```python
from build123d import *

# Parameters (mm, degrees)
SKETCH1_W           = 140
SKETCH1_H           = 205
SKETCH1_R           = 2.125
BOSS_EXTRUDE1_DEPTH = 3.175
SKETCH2_R           = 2.125
CUT_EXTRUDE1_DEPTH  = 125.162516989


with BuildPart() as part:
    # Sketch1 → Boss-Extrude1 (new body)
    with BuildSketch(Plane.XY):
        Rectangle(SKETCH1_W, SKETCH1_H)
        with Locations((0, 91.5)):
            Circle(SKETCH1_R, mode=Mode.SUBTRACT)
        with Locations((25.11473671, 48)):
            Circle(SKETCH1_R, mode=Mode.SUBTRACT)
        with Locations((-25.11473671, 48)):
            Circle(SKETCH1_R, mode=Mode.SUBTRACT)
        with Locations((0, 62.5)):
            Circle(SKETCH1_R, mode=Mode.SUBTRACT)
        with Locations((-62, -94.5)):
            Circle(SKETCH1_R, mode=Mode.SUBTRACT)
        with Locations(Location((-38, -94.5, 0), (0, 0, 180))):
            Circle(SKETCH1_R, mode=Mode.SUBTRACT)
        with Locations((-38, -70.5)):
            Circle(SKETCH1_R, mode=Mode.SUBTRACT)
        with Locations(Location((-62, -70.5, 0), (0, 0, 180))):
            Circle(SKETCH1_R, mode=Mode.SUBTRACT)
        with Locations((38, -94.5)):
            Circle(SKETCH1_R, mode=Mode.SUBTRACT)
        with Locations(Location((62, -94.5, 0), (0, 0, 180))):
            Circle(SKETCH1_R, mode=Mode.SUBTRACT)
        with Locations((62, -70.5)):
            Circle(SKETCH1_R, mode=Mode.SUBTRACT)
        with Locations(Location((38, -70.5, 0), (0, 0, 180))):
            Circle(SKETCH1_R, mode=Mode.SUBTRACT)
    extrude(amount=BOSS_EXTRUDE1_DEPTH)

    # Sketch2 → Cut-Extrude1 (cut, through all)
    with BuildSketch(Plane.XY.offset(3.175)):
        with Locations((-62, 94.5)):
            Circle(SKETCH2_R)
        with Locations((-62, 60.5)):
            Circle(SKETCH2_R)
        with Locations((-62, 26.5)):
            Circle(SKETCH2_R)
        with Locations((-62, -7.5)):
            Circle(SKETCH2_R)
        with Locations((-28, 26.5)):
            Circle(SKETCH2_R)
        with Locations((-28, -7.5)):
            Circle(SKETCH2_R)
        with Locations(Location((28, -7.5, 0), (0, 0, 180))):
            Circle(SKETCH2_R)
        with Locations(Location((28, 26.5, 0), (0, 0, 180))):
            Circle(SKETCH2_R)
        with Locations(Location((62, -7.5, 0), (0, 0, 180))):
            Circle(SKETCH2_R)
        with Locations(Location((62, 26.5, 0), (0, 0, 180))):
            Circle(SKETCH2_R)
        with Locations(Location((62, 60.5, 0), (0, 0, 180))):
            Circle(SKETCH2_R)
        with Locations(Location((62, 94.5, 0), (0, 0, 180))):
            Circle(SKETCH2_R)
    extrude(amount=-CUT_EXTRUDE1_DEPTH, mode=Mode.SUBTRACT)


solid = part.part
```
Part model, mm, in its own coordinate system. Round coordinates to 2 decimals unless told otherwise and drop trailing zeros. Order: outer loops, then holes, each group sorted by start corner. A loop starts at its lowest first (then second) coordinate and runs counter-clockwise, first axis right, second up. Notation, with made-up numbers: M 19.25,42 L 55.25,42 A34 cw 55.25,75 Z; hole C 77,47.5 d4. An arc over 180 degrees is marked long. Put each result on its own line as item: value. Start each with the question number.
1. Slice it at C-C on y = -7.5. List the corners of the cut face in (x, z) (3 decimals), then the cut area to 3 significant figures.
2. Drop a flat-ended pin along its axis: pin 1 (2.5 mm diameter, centred on x = -62, y = -70.5, fed in from +Z). Give the stop position or say it passes through.
3. Drill centre lines: probe 1 along Y at (x, z) = (-28, 1.95) (3 decimals); probe 2 along X at (y, z) = (59, 2.55); probe 3 along X at (y, z) = (63.5, 1.5) (3 decimals). Where is each one in solid material? Low to high. Write a range as [from, to].
4. Slice it at D-D on x = -38. List the corners of the cut face in (y, z) (3 decimals), then the cut area to 3 significant figures.
5. Slice it at B-B on x = -62. List the corners of the cut face in (y, z) (3 decimals).
6. Slice it at A-A on y = 48. List the corners of the cut face in (x, z) (3 decimals).
Findings:
1. outline: M -70,0 L -64.125,0 L -64.125,3.175 L -70,3.175 Z; M -59.875,0 L -30.125,0 L -30.125,3.175 L -59.875,3.175 Z; M -25.875,0 L 25.875,0 L 25.875,3.175 L -25.875,3.175 Z; M 30.125,0 L 59.875,0 L 59.875,3.175 L 30.125,3.175 Z; M 64.125,0 L 70,0 L 70,3.175 L 64.125,3.175 Z
1. area: 391 mm2
2. pin 1: through
3. probe 1: [-102.5, -9.625], [-5.375, 24.375], [28.625, 102.5]
3. probe 2: [-70, -63.51], [-60.49, 60.49], [63.51, 70]
3. probe 3: [-70, -1.875], [1.875, 70]
4. outline: M -102.5,0 L -96.625,0 L -96.625,3.175 L -102.5,3.175 Z; M -92.375,0 L -72.625,0 L -72.625,3.175 L -92.375,3.175 Z; M -68.375,0 L 102.5,0 L 102.5,3.175 L -68.375,3.175 Z
4. area: 624 mm2
5. outline: M -102.5,0 L -96.625,0 L -96.625,3.175 L -102.5,3.175 Z; M -92.375,0 L -72.625,0 L -72.625,3.175 L -92.375,3.175 Z; M -68.375,0 L -9.625,0 L -9.625,3.175 L -68.375,3.175 Z; M -5.375,0 L 24.375,0 L 24.375,3.175 L -5.375,3.175 Z; M 28.625,0 L 58.375,0 L 58.375,3.175 L 28.625,3.175 Z; M 62.625,0 L 92.375,0 L 92.375,3.175 L 62.625,3.175 Z; M 96.625,0 L 102.5,0 L 102.5,3.175 L 96.625,3.175 Z
6. outline: M -70,0 L -27.24,0 L -27.24,3.175 L -70,3.175 Z; M -22.99,0 L 22.99,0 L 22.99,3.175 L -22.99,3.175 Z; M 27.24,0 L 70,0 L 70,3.175 L 27.24,3.175 Z
